Autodesk Fusion 360 part; units mm, degrees
sketch "Sketch1" plane through (0, 0, 0) normal (0, 0, 1) x (1, 0, 0)
  line L0 (0, 0) -> (90, 0)
  line L1 (90, 0) -> (90, 50)
  line L2 (90, 50) -> (0, 50)
  line L3 (0, 50) -> (0, 0)
  line L4 (-2, -2) -> (92, -2)
  line L5 (92, -2) -> (92, 52)
  line L6 (92, 52) -> (-2, 52)
  line L7 (-2, 52) -> (-2, -2)
  line L8 (-5, -5) -> (95, -5)
  line L9 (95, -5) -> (95, 55)
  line L10 (95, 55) -> (-5, 55)
  line L11 (-5, 55) -> (-5, -5)
  line L12 (30, 0) -> (60, 0)
  line L13 (60, 0) -> (60, -2)
  line L14 (60, -2) -> (30, -2)
  line L15 (30, -2) -> (30, 0)
  dimension "d1" = 90
  dimension "d2" = 50
  dimension "d3" = 2
  dimension "d4" = 5
  dimension "d5" = 30
extrude "Extrude1" add sketch "Sketch1" along normal blind 55 contours L0 L1 L2 L3 L4 L5 L6 L7 L13 L15
extrude "Extrude2" add sketch "Sketch1" against normal blind 3 contours L0 L1 L2 L3 L12 | L0 L1 L2 L3 L4 L5 L6 L7 L13 L15 | L0 L4 L12 L13 L14 L15 | L8 L9 L10 L11
fillet "Fillet1" radius 15 2 edges at (30, -1, 55) (60, -1, 55)
fillet "Fillet2" radius 3 4 edges at (-5, -5, -1.5) (95, -5, -1.5) (95, 55, -1.5) (-5, 55, -1.5)
fillet "Fillet3" radius 2 4 edges at (92, -2, 27.5) (92, 52, 27.5) (-2, -2, 27.5) (-2, 52, 27.5)
fillet "Fillet4" radius 0.5 13 edges at (30, -2, 20) (25.6066, -2, 50.6066) (7.5, -2, 55) (-1.4142, -1.4142, 55) (-2, 25, 55) (-1.4142, 51.4142, 55) (45, 52, 55) (91.4142, 51.4142, 55) (92, 25, 55) (91.4142, -1.4142, 55) (82.5, -2, 55) (64.3934, -2, 50.6066) (60, -2, 20)
fillet "Fillet5" radius 1 8 edges at (94.1213, -4.1213, 0) (95, 25, 0) (94.1213, 54.1213, 0) (45, 55, 0) (-4.1213, 54.1213, 0) (-5, 25, 0) (-4.1213, -4.1213, 0) (45, -5, 0)
equation "d1 = base_width"
equation "d2 = base_depth"
equation "d3 = wall_thickness"
equation "d4 = wall_thickness + base_overhang"
equation "d5 = base_width / 3"
equation "d6 = wall_height"
equation "d8 = -( wall_thickness + 1 mm )"
equation "base_width = 90 mm"
equation "base_depth = 50 mm"
equation "wall_height = 55 mm"
equation "wall_thickness = 2 mm"
equation "base_overhang = 3 mm"
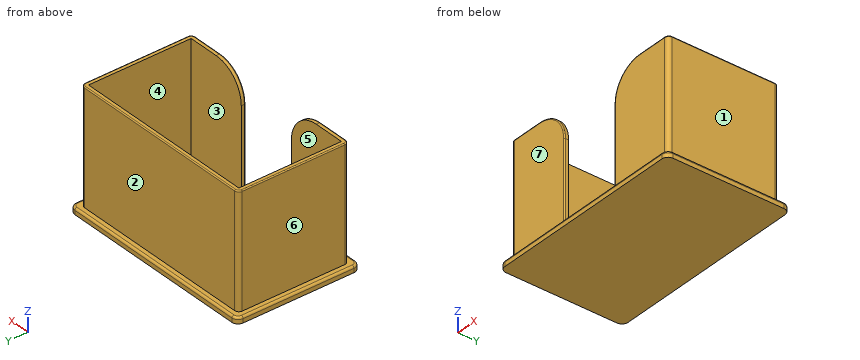
Geometry check sheet. Reference: the model listing, model coordinates, mm. Face numbers are marked on the shaded views. A direction names the side the tool comes from. Round coordinates to 2 decimals unless told otherwise and drop trailing zeros. Write each loop counter-clockwise with the first axis right and the second up, starting at its lowest first coordinate (ties: lowest second). Pieces come first, ordered by that corner, then holes. Notation, with made-up numbers: (4.5, -11) -> (8.5, -11) arc R21 ccw to (8.5, -4) -> close; hole circle Ø2 at (14, 33). An arc over 180 degrees is marked (long way). Put each result on its own line as item: value.
1) Cross-section at D-D, the plane x = 84. Enter the section's corners in (y, z).
Recorded:
outline: (-5, -3) -> (55, -3) -> (55, -1) arc R1 ccw to (54, 0) -> (52, 0) -> (52, 54.5) arc R0.5 ccw to (51.5, 55) -> (50, 55) -> (50, 0) -> (0, 0) -> (0, 55) -> (-1.5, 55) arc R0.5 ccw to (-2, 54.5) -> (-2, 0) -> (-4, 0) arc R1 ccw to (-5, -1) -> close
2) Thickness scan on probe 1 along X at (y, z) = (48, 37); probe 2 along Y at (x, z) = (11.5, 43.5); probe 3 along Y at (x, z) = (51.5, 48). Record the ranges inside material, lowest first. Write a range as from..to.
Recorded:
probe 1: x = -2..0, 90..92
probe 2: y = -2..0, 50..52
probe 3: y = 50..52
3) Cross-section at B-B, the plane x = 55. Enter the section's corners in (y, z), plus the area to 3 significant figures.
Recorded:
outline: (-5, -3) -> (55, -3) -> (55, -1) arc R1 ccw to (54, 0) -> (52, 0) -> (52, 54.5) arc R0.5 ccw to (51.5, 55) -> (50, 55) -> (50, 0) -> (-4, 0) arc R1 ccw to (-5, -1) -> close
area: 290 mm2
4) Access from +Z, -Z, +X, -X, +Y, -Y to the whole of each face (thin tool, end or side, straight path). Record for the marked faces 5, 6 and 7.
Recorded:
face 5: +Z
face 6: +Z, -X, +Y, -Y
face 7: +Z, +X, -X, -Y
5) Cross-section at A-A, the plane y = 4. Enter the section's corners in (x, z), plus the area to 3 significant figures.
Recorded:
outline: (-5, -3) -> (95, -3) -> (95, -1) arc R1 ccw to (94, 0) -> (92, 0) -> (92, 54.5) arc R0.5 ccw to (91.5, 55) -> (90, 55) -> (90, 0) -> (0, 0) -> (0, 55) -> (-1.5, 55) arc R0.5 ccw to (-2, 54.5) -> (-2, 0) -> (-4, 0) arc R1 ccw to (-5, -1) -> close
area: 519 mm2
6) Depth check by flat-ended pin: P1, Ø3, axis at x = 66, y = 33, coming from the +Z side; P2, Ø8, axis at x = 48, z = 30, coming from the -Y side; P3, Ø1, axis at x = 77, z = 40, coming from the -Y side. Enter the tip coordinate at first touch or a pass-through.
Recorded:
P1: stops at z = 0
P2: stops at y = 50
P3: stops at y = -2
7) Cross-section at C-C, the plane z = 14.5. Enter the section's corners in (x, y).
Recorded:
outline: (-2, 0) arc R2 ccw to (0, -2) -> (29.5, -2) arc R0.5 ccw to (30, -1.5) -> (30, 0) -> (0, 0) -> (0, 50) -> (90, 50) -> (90, 0) -> (60, 0) -> (60, -1.5) arc R0.5 ccw to (60.5, -2) -> (90, -2) arc R2 ccw to (92, 0) -> (92, 50) arc R2 ccw to (90, 52) -> (0, 52) arc R2 ccw to (-2, 50) -> close
8) Release check for a two-part mould opening along X. For the marked faces 1, 2, 3 and 4 record: pulls with the +X half, pulls with the -X half, needs draft (parallel to the pull), parting line crosses it, or undercut.
Recorded:
face 1: pulls with the +X half
face 2: needs draft
face 3: undercut
face 4: undercut
